from build123d import *

# Parameters (mm, degrees)
SKETCH_1_R           = 5
EXTRUDE_1_DEPTH      = 21
EXTRUDE_2_DEPTH      = 4
SKETCH_3_R           = 4
EXTRUDE_3_DEPTH      = 1
SKETCH_4_R           = 2.5
EXTRUDE_4_DEPTH      = 7
SKETCH_5_R           = 4
EXTRUDE_5_DEPTH      = 4
SKETCH_6_R           = 5.5
EXTRUDE_6_DEPTH      = 3
SKETCH_7_R           = 7
SKETCH_7_R_2         = 5
EXTRUDE_7_DEPTH      = 12
SKETCH_9_W           = 9.328895196
SKETCH_9_H           = 0.721756852
CUT_EXTRUDE_9_DEPTH  = 1.5
SKETCH_10_R          = 4.2723733
CUT_EXTRUDE_10_DEPTH = 19


with BuildPart() as part:
    # Sketch 1 → Extrude 1 (new body)
    with BuildSketch(Plane(origin=(0, 0, 0), x_dir=(1, 0, 0), z_dir=(0, 1, 0))):
        with Locations(Location((0, 0, 0), (0, 0, 90))):
            Circle(SKETCH_1_R)
    extrude(amount=EXTRUDE_1_DEPTH)

    # Sketch 2 → Extrude 2 (add)
    with BuildSketch(Plane(origin=(0, 21, 0), x_dir=(1, 0, 0), z_dir=(0, 1, 0))):
        Polygon((5.132313302, 4.653961771), (-1.464292471, 6.771694586), (-6.596605773, 2.117732814), (-5.132313302, -4.653961771), (1.464292471, -6.771694586), (6.596605773, -2.117732814), align=None)
    extrude(amount=EXTRUDE_2_DEPTH)

    # Sketch 3 → Extrude 3 (add)
    with BuildSketch(Plane(origin=(0, 25, 0), x_dir=(1, 0, 0), z_dir=(0, 1, 0))):
        with Locations(Location((0, 0, 0), (0, 0, 270))):
            Circle(SKETCH_3_R)
    extrude(amount=EXTRUDE_3_DEPTH)

    # Sketch 4 → Extrude 4 (add)
    with BuildSketch(Plane(origin=(0, 26, 0), x_dir=(1, 0, 0), z_dir=(0, 1, 0))):
        with Locations(Location((0, 0, 0), (0, 0, 270))):
            Circle(SKETCH_4_R)
    extrude(amount=EXTRUDE_4_DEPTH)

    # Sketch 5 → Extrude 5 (add)
    with BuildSketch(Plane(origin=(0, 33, 0), x_dir=(1, 0, 0), z_dir=(0, 1, 0))):
        with Locations(Location((0, 0, 0), (0, 0, 270))):
            Circle(SKETCH_5_R)
    extrude(amount=EXTRUDE_5_DEPTH)

    # Sketch 6 → Extrude 6 (add)
    with BuildSketch(Plane(origin=(0, 28, 0), x_dir=(-1, 0, 0), z_dir=(0, 1, 0))):
        with Locations(Location((0, 0, 0), (0, 0, 90))):
            Circle(SKETCH_6_R)
    extrude(amount=EXTRUDE_6_DEPTH)



with BuildPart() as body_2:
    # Sketch 7 → Extrude 7 (new body)
    with BuildSketch(Plane.XZ.offset(-21)):
        with Locations(Location((0, 0, 0), (0, 0, 270))):
            Circle(SKETCH_7_R)
        with Locations(Location((0, 0, 0), (0, 0, 270))):
            Circle(SKETCH_7_R_2, mode=Mode.SUBTRACT)
    extrude(amount=EXTRUDE_7_DEPTH)


with BuildPart() as part_1:
    add(part.part)

    add(body_2.part)  # Revolve 1 merges body 2
    # Sketch 8 → Revolve 1 (revolve)
    with BuildSketch(Plane(origin=(0, 0, 0), x_dir=(0, 0, -1), z_dir=(1, 0, 0)), mode=Mode.PRIVATE) as revolve_1_sk:
        Polygon((3.877064073, 18.84702899), (3.877064073, 20), (5.073285263, 20), (8.5, 20), (10, 21.5), (20, 21.5), (20, 20.988021683), (21.3, 20.988021683), (21.3, 21.5), (22.180246255, 21.5), (22.180246255, 20), (11.774720378, 20), (9.998528163, 18.84702899), align=None)
    revolve(revolve_1_sk.sketch.rotate(Axis((0, 15, 0), (0, 0, -1)), 90), axis=Axis((0, 15, 0), (0, 0, -1)))

    # Sketch 9 → Cut-Extrude 9 (cut)
    with BuildSketch(Plane(origin=(0, 37, 0), x_dir=(1, 0, 0), z_dir=(0, 1, 0))):
        Rectangle(SKETCH_9_W, SKETCH_9_H)
    extrude(amount=-CUT_EXTRUDE_9_DEPTH, mode=Mode.SUBTRACT)

    # Sketch 10 → Cut-Extrude 10 (cut)
    with BuildSketch(Plane.XZ):
        with Locations(Location((0, 0, 0), (0, 0, 270))):
            Circle(SKETCH_10_R)
    extrude(amount=-CUT_EXTRUDE_10_DEPTH, mode=Mode.SUBTRACT)


solid = part_1.part
Build history of the part. All positions in model axes, mm. A direction names the side the tool comes from. Round coordinates to 2 decimals unless told otherwise and drop trailing zeros. Loops run counter-clockwise (first coordinate to the right, second up) from the corner with the lowest first, then second, coordinate; pieces in that order, holes last. Notation, with made-up numbers: (83, 33.25) -> (94, 33.25) arc R17 ccw to (94, 40.25) -> close; hole circle Ø4 at (-26, 86). An arc over 180 degrees is marked (long way). Answer in a Markdown table with one row per item.
Item 1: Saw through at D-D (y = 5.5). Write the cut outline in (x, z), and give its area (3 significant figures).
Answers below:
| item | result |
|---|---|
| outline | circle Ø10 at (0, 0); hole circle Ø8.54 at (0, 0) |
| area | 21.2 mm² |
Item 2: Saw through at A-A (y = 15). Write the cut outline in (x, z), and give its area (3 significant figures).
Answers below:
| item | result |
|---|---|
| outline | (-6.5, -22.18) -> (-5, -22.18) -> (-5, -11.77) -> (-3.85, -10) -> (-3.85, -5.85) arc R7 ccw to (3.85, -5.85) -> (3.85, -10) -> (5, -11.77) -> (5, -22.18) -> (6.5, -22.18) -> (6.5, -21.3) -> (5.99, -21.3) -> (5.99, -20) -> (6.5, -20) -> (6.5, -10) -> (5, -8.5) -> (5, -4.9) arc R7 ccw (long way) to (-5, -4.9) -> (-5, -8.5) -> (-6.5, -10) -> (-6.5, -20) -> (-5.99, -20) -> (-5.99, -21.3) -> (-6.5, -21.3) -> close; hole circle Ø8.54 at (0, 0) |
| area | 147 mm² |
Item 3: Mould opens along X. For faces 1 (the cylindrical face through (-1.298, 20.846, -20.659)), 2 (the cylindrical face through (1.283, 9.367, -4.075)), 3 (the flat face through (0, 31, -3)) say: +X half, -X half, draft (parallel to the pull), parting line (faces both ways), or undercut.
Answers below:
| item | result |
|---|---|
| face 1 | parting line |
| face 2 | undercut |
| face 3 | draft |
Item 4: Saw through at C-C (y = 24). Write the cut outline in (x, z).
Answers below:
| item | result |
|---|---|
| outline | (-6.6, -2.12) -> (-1.46, -6.77) -> (5.13, -4.65) -> (6.6, 2.12) -> (1.46, 6.77) -> (-5.13, 4.65) -> close |
Item 5: Which spindle directions (+Z, -Z, +X, -X, +Y, -Y) get a long thin tool onto all of the face, cutting with end or side? Do faces 4 (the flat face through (0, 28, -3)), 5 (the cylindrical face through (-5.37, 29.48, -1.19)), 6 (the flat face through (5, 9, 2)), 7 (the cylindrical face through (-1.08, 19.88, -16.9)). Say none if no direction does.
Answers below:
| item | result |
|---|---|
| face 4 | none |
| face 5 | +Y |
| face 6 | -Y |
| face 7 | -Z |
Item 6: Saw through at B-B (z = -15.75). Write the cut outline in (x, y), and give its area (3 significant figures).
Answers below:
| item | result |
|---|---|
| outline | circle Ø13 at (0, 15); hole circle Ø10 at (0, 15) |
| area | 54.2 mm² |
Item 7: Pin check, flat tips, straight feed: pin 1 (4 mm diameter, centred on x = -2.5, y = 17, fed in from +Z); pin 2 (1.5 mm diameter, centred on x = 1.5, z = -14, fed in from -Y); pin 3 (4 mm diameter, centred on y = 17.5, z = -11, fed in from +X). Stop position of each tip, or through.
Answers below:
| item | result |
|---|---|
| pin 1 | stops at z = 6.98 |
| pin 2 | stops at y = 8.54 |
| pin 3 | stops at x = 6.48 |
Item 8: Drill centre lines: L1, parallel to Y at x = 0.75, z = -3.5; L2, parallel to X at y = 15, z = -19; L3, parallel to Y at x = 1.5, z = -3.75. Where is each one in solid material? Low to high. Write a range as [from, to].
Answers below:
| item | result |
|---|---|
| L1 | y = [19, 26], [28, 31], [33, 37] |
| L2 | x = [-6.5, -5], [5, 6.5] |
| L3 | y = [19, 25], [28, 31] |
